```python
from build123d import *

# Parameters (mm, degrees)
F1_DEPTH = 300
F2_R     = 50
F3_DEPTH = 70.156318
F4_R     = 80
F5_DEPTH = 70.156318
F6_W     = 200
F6_H     = 150
F7_DEPTH = 500.001


with BuildPart() as f1:
    # F0 (on Front) → F1 (new body)
    with BuildSketch(Plane.XZ):
        Polygon((-250, -250), (250, -250), (250, 125), (125, 250), (-125, 250), (-250, 125), align=None)
        with BuildLine():
            ThreePointArc((165.359457, 112.5), (191.143783, 58.856217), (200, 0))
            ThreePointArc((200, 0), (191.143783, -58.856217), (165.359457, -112.5))
            ThreePointArc((165.359457, -112.5), (148.99364, -133.419995), (130, -151.986842))
            ThreePointArc((130, -151.986842), (109.63833, -167.270549), (87.5, -179.843682))
            ThreePointArc((87.5, -179.843682), (0, -200), (-87.5, -179.843682))
            ThreePointArc((-87.5, -179.843682), (-109.63833, -167.270549), (-130, -151.986842))
            ThreePointArc((-130, -151.986842), (-148.99364, -133.419995), (-165.359457, -112.5))
            ThreePointArc((-165.359457, -112.5), (-200, 0), (-165.359457, 112.5))
            ThreePointArc((-165.359457, 112.5), (-148.99364, 133.419995), (-130, 151.986842))
            ThreePointArc((-130, 151.986842), (-109.63833, 167.270549), (-87.5, 179.843682))
            ThreePointArc((-87.5, 179.843682), (0, 200), (87.5, 179.843682))
            ThreePointArc((87.5, 179.843682), (109.63833, 167.270549), (130, 151.986842))
            ThreePointArc((130, 151.986842), (148.99364, 133.419995), (165.359457, 112.5))
        make_face(mode=Mode.SUBTRACT)
        with BuildLine():
            Line((-130, 112.5), (-130, 151.986842))
            ThreePointArc((-130, 151.986842), (-148.99364, 133.419995), (-165.359457, 112.5))
            Line((-165.359457, 112.5), (-130, 112.5))
        make_face()
        with BuildLine():
            Line((-87.5, 179.843682), (87.5, 179.843682))
            ThreePointArc((87.5, 179.843682), (0, 200), (-87.5, 179.843682))
        make_face()
        with BuildLine():
            Line((130, 112.5), (165.359457, 112.5))
            ThreePointArc((165.359457, 112.5), (148.99364, 133.419995), (130, 151.986842))
            Line((130, 151.986842), (130, 112.5))
        make_face()
        with BuildLine():
            ThreePointArc((130, -151.986842), (148.99364, -133.419995), (165.359457, -112.5))
            Line((165.359457, -112.5), (130, -112.5))
            Line((130, -112.5), (130, -151.986842))
        make_face()
        with BuildLine():
            ThreePointArc((-87.5, -179.843682), (0, -200), (87.5, -179.843682))
            Line((87.5, -179.843682), (-87.5, -179.843682))
        make_face()
        with BuildLine():
            ThreePointArc((-165.359457, -112.5), (-148.99364, -133.419995), (-130, -151.986842))
            Line((-130, -151.986842), (-130, -112.5))
            Line((-130, -112.5), (-165.359457, -112.5))
        make_face()
    extrude(amount=F1_DEPTH)

    # F2 (on face) → F3 (cut, through all)
    with BuildSketch(Plane.XY.offset(250)):
        with Locations((0, -150)):
            Circle(F2_R)
    extrude(amount=-F3_DEPTH, mode=Mode.SUBTRACT)

    # F4 (on face) → F5 (cut, through all)
    with BuildSketch(Plane(origin=(0, 0, -250), x_dir=(1, 0, 0), z_dir=(0, 0, -1))):
        with Locations((0, 150)):
            Circle(F4_R)
    extrude(amount=-F5_DEPTH, mode=Mode.SUBTRACT)

    # F6 (on face) → F7 (cut, through all)
    with BuildSketch(Plane.YZ.offset(250)):
        with Locations((-150, 0)):
            Rectangle(F6_W, F6_H)
    extrude(amount=-F7_DEPTH, mode=Mode.SUBTRACT)


solid = f1.part
```
Design review of the part built by this model. Coordinates are the model's own, in mm. A direction names the side the tool comes from. Coordinates: 2 decimals unless noted, no trailing zeros. Order: outer loops, then holes, each group sorted by start corner. A loop starts at its lowest first (then second) coordinate and runs counter-clockwise, first axis right, second up.
1) Mouldability with a two-part tool opening along X and no side actions: class faces 1 (the flat face through (-224, -50, -1)), 2 (the flat face through (-250, -148, -102)), 3 (the flat face through (250, -148, -107)), 4 (the flat face through (-130, -148, -133)) as +X half, -X half, draft (parallel to the pull), parting line (faces both ways), or undercut.
2) For faces 5 (the cylindrical face through (-10.41, -229.32, -215.41)), 6 (the flat face through (225, -50, -1)), 7 (the flat face through (-147, -148, -112.5)), list the 3-axis set-ups (+Z, -Z, +X, -X, +Y, -Y) from which the entire face can be reached by the end or side of a thin tool; tool diameter is ignored.
3) Take a section at A-A, the plane x = 0. Give the boundary of the cut face in (y, z).
4) Take a section at B-B, the plane y = -272. Give the boundary of the cut face in (x, z).
5) Clearance check with flat-ended pins moving along their axes: pin 1 (1 mm diameter, centred on x = 191, y = -97.5, fed in from +Z); pin 2 (12 mm diameter, centred on y = -173.5, z = 134.5, fed in from +X); pin 3 (12 mm diameter, centred on y = -193.5, z = 133.5, fed in from -X). State where each tip first meets the part, or that it passes through.
6) Wall thickness on line 1 along Y through (x, z) = (205, 11); line 2 along Y through (x, z) = (0, 216); line 3 along Z through (x, y) = (53.5, -87): over which ranges is each line inside the solid? List them lowest first.
7) Take a section at C-C, the plane z = 162. Give the boundary of the cut face in (x, y), and give its area (3 significant figures).
Returned:
1. face 1: draft
1. face 2: -X half
1. face 3: +X half
1. face 4: undercut
2. face 5: -Z
2. face 6: +X, -X
2. face 7: +Y, -Y
3. outline: (-300, -250) - (-230, -250) - (-230, -179.84) - (-300, -179.84) - close; (-300, 179.84) - (-200, 179.84) - (-200, 250) - (-300, 250) - close; (-100, 179.84) - (0, 179.84) - (0, 250) - (-100, 250) - close; (-70, -250) - (0, -250) - (0, -179.84) - (-70, -179.84) - close
4. outline: (-250, -250) - (250, -250) - (250, 125) - (125, 250) - (-125, 250) - (-250, 125) - close; hole (-165.36, -112.5) - (-130, -112.5) - (-130, -151.99) arc R200 ccw to (-87.5, -179.84) - (87.5, -179.84) arc R200 ccw to (130, -151.99) - (130, -112.5) - (165.36, -112.5) arc R200 ccw to (200, 0) arc R200 ccw to (165.36, 112.5) - (130, 112.5) - (130, 151.99) arc R200 ccw to (87.5, 179.84) - (-87.5, 179.84) arc R200 ccw to (-130, 151.99) - (-130, 112.5) - (-165.36, 112.5) arc R200 ccw to start
5. pin 1: stops at z = 184.5
5. pin 2: stops at x = 246.5
5. pin 3: stops at x = -247.5
6. line 1: y = -300 to -250, -50 to 0
6. line 2: y = -300 to -200, -100 to 0
6. line 3: z = -250 to -179.84, 179.84 to 250
7. outline: (-213, -300) - (-117.29, -300) - (-117.29, 0) - (-213, 0) - close; (117.29, -300) - (213, -300) - (213, 0) - (117.29, 0) - close
7. area: 57,400 mm2
